```python
from build123d import *

# Parameters (mm, degrees)
SKETCH_W                        = 15
SKETCH_H                        = 25
PAD_DEPTH                       = 6
POCKET_DEPTH                    = 3
SKETCH002_R                     = 2.5
POCKET001_DEPTH                 = 3
SKETCH003_R                     = 1.5
POCKET002_DEPTH                 = 6.001
SKETCH004_R                     = 2
POCKET003_DEPTH                 = 1.5
SKETCH005_R                     = 1.5
POCKET004_DEPTH                 = 65.532504
SKETCH005_LINEARPATTERN_2_R     = 1.5
POCKET004_LINEARPATTERN_2_DEPTH = 65.532504
LINEARPATTERN001_COUNT          = 2
LINEARPATTERN001_PITCH          = 19
HOLE_D                          = 3
HOLE_DEPTH                      = 25
HOLE_CBORE_D                    = 5
HOLE_CBORE_DEPTH                = 1.5
FILLET_R                        = 1


with BuildPart() as part:
    # Sketch → Pad (new body)
    with BuildSketch(Plane.XY):
        Rectangle(SKETCH_W, SKETCH_H)
    extrude(amount=PAD_DEPTH)

    # Sketch001 (on Face6 of Pad) → Pocket (cut)
    with BuildSketch(Plane.XY.offset(6)):
        with BuildLine():
            Line((4, 4), (4, -4))
            ThreePointArc((-4, -4), (0, -8), (4, -4))
            Line((-4, -4), (-4, 4))
            ThreePointArc((4, 4), (0, 8), (-4, 4))
        make_face()
    extrude(amount=-POCKET_DEPTH, mode=Mode.SUBTRACT)

    # Sketch002 (on Face4 of Pocket) → Pocket001 (cut)
    with BuildSketch(Plane(origin=(0, 0, 0), x_dir=(1, 0, 0), z_dir=(0, 0, -1))):
        with Locations((4, 0)):
            Circle(SKETCH002_R)
    extrude(amount=-POCKET001_DEPTH, mode=Mode.SUBTRACT)

    # Sketch003 (on Face5 of Pocket001) → Pocket002 (cut, through all)
    with BuildSketch(Plane.XY.offset(6)):
        with Locations((4, 0)):
            Circle(SKETCH003_R)
    extrude(amount=-POCKET002_DEPTH, mode=Mode.SUBTRACT)

    # Sketch004 (on Face14 of Pocket002) → Pocket003 (cut)
    with BuildSketch(Plane.XY.offset(3)):
        with Locations((0, -4)):
            Circle(SKETCH004_R)
    extrude(amount=-POCKET003_DEPTH, mode=Mode.SUBTRACT)

    # Sketch005 (on Face5 of Pocket003) → Pocket004 (cut, through all)
    with BuildSketch(Plane.XY.offset(6)):
        with Locations((-4.5, 9.5)):
            Circle(SKETCH005_R)
    pocket004 = extrude(amount=-POCKET004_DEPTH, mode=Mode.SUBTRACT)

    # Sketch005 LinearPattern 2 → Pocket004 LinearPattern 2 (cut, through all)
    with BuildSketch(Plane(origin=(9, 0, 6), x_dir=(1, 0, 0), z_dir=(0, 0, 1))):
        with Locations((-4.5, 9.5)):
            Circle(SKETCH005_LINEARPATTERN_2_R)
    pocket004_linearpattern_2 = extrude(amount=-POCKET004_LINEARPATTERN_2_DEPTH, mode=Mode.SUBTRACT)

    # LinearPattern001: Pocket004, Pocket004 LinearPattern 2 ×2
    with Locations(*[(0, -i * LINEARPATTERN001_PITCH, 0) for i in range(1, LINEARPATTERN001_COUNT)]):
        add(pocket004, mode=Mode.SUBTRACT)
        add(pocket004_linearpattern_2, mode=Mode.SUBTRACT)

    # Hole
    with Locations(Plane(origin=(-7.5, 0, 0), x_dir=(0, -1, 0), z_dir=(-1, 0, 0))):
        with Locations((0, 3)):
            CounterBoreHole(HOLE_D / 2, HOLE_CBORE_D / 2, HOLE_CBORE_DEPTH, depth=HOLE_DEPTH)

    # Fillet
    fillet_edges = [part.edges().sort_by_distance(p)[0] for p in [
        (-7.5, -12.5, 3),
        (7.5, -12.5, 3),
        (-7.5, 12.5, 3),
        (7.5, 12.5, 3),
    ]]
    fillet(fillet_edges, radius=FILLET_R)


solid = part.part
```
Can you work these out from the model? Positions are in its coordinate system, mm. A direction names the side the tool comes from. Coordinates: 2 decimals unless noted, no trailing zeros. Loops run counter-clockwise (first coordinate to the right, second up) from the corner with the lowest first, then second, coordinate; pieces in that order, holes last.
Item 1: Suppose I cut it at B-B (x = -4.5). Please give me the cut outline in (y, z).
Answers below:
outline: (-12.5, 0) - (-11, 0) - (-11, 6) - (-12.5, 6) - close; (-8, 0) - (8, 0) - (8, 6) - (-8, 6) - close; (11, 0) - (12.5, 0) - (12.5, 6) - (11, 6) - close; hole circle Ø3 at (0, 3)
Item 2: Suppose I cut it at C-C (z = 3.5). State how many separate pieces and enclosed holes the cut face has, then the cut area to 3 significant figures.
Answers below:
separate pieces: 2
enclosed holes: 4
area: 209 mm2
Item 3: Suppose I cut it at A-A (y = -9.5). Please give me the cut outline in (x, z), then the cut area to 3 significant figures.
Answers below:
outline: (-7.5, 0) - (-6, 0) - (-6, 6) - (-7.5, 6) - close; (-3, 0) - (3, 0) - (3, 6) - (-3, 6) - close; (6, 0) - (7.5, 0) - (7.5, 6) - (6, 6) - close
area: 54.0 mm2
Item 4: Which directions (+Z, -Z, +X, -X, +Y, -Y) give clear straight access to the entire face, cutting with the end or side of a thin tool? Please do faces 5 (the face through (-2.833, -0.325, 1.536)), 6 (the face through (5, -2, 3)), 7 (the face through (5.5, 0, 4.9)), 8 (the face through (-7.215, -12.199, 3.042)), 9 (the face through (0, 5, 3)).
Answers below:
face 5: +X, -X
face 6: -Z
face 7: +Z, -Z
face 8: +Z, -Z, -X, -Y
face 9: +Z
Item 5: Please list where these lines run through material, in increasing order: L1, parallel to Y at x = 4.5, z = 4.2; L2, parallel to Y at x = -3.25, z = 2; L3, parallel to X at y = 2, z = 2.75.
Answers below:
L1: y = -12.5 to -11, -8 to -1.41, 1.41 to 8, 11 to 12.5
L2: y = -12.5 to -10.33, -8.67 to -1.12, 1.12 to 8.67, 10.33 to 12.5
L3: x = -6 to 2.5, 5.5 to 7.5
Item 6: I'm going to push flat-ended pins straight in: pin 1 (2 mm diameter, centred on x = 0, y = -4.5, fed in from +Z); pin 2 (4.5 mm diameter, centred on x = 0, y = -4, fed in from +Z). Where does each tip first touch, or does it pass through?
Answers below:
pin 1: stops at z = 1.5
pin 2: stops at z = 3
Item 7: If we mould it in two halves opening along Y, with no side actions, what happens to faces 1 (the face through (0, 12.5, 3)), 2 (the face through (6.163, -0.195, 4.487)), 3 (the face through (-7.5, -3, 3)), 4 (the face through (4, 3, 5))? For each: released by +Y, released by -Y, zero draft, split by the parting line, or undercut.
Answers below:
face 1: released by +Y
face 2: undercut
face 3: zero draft
face 4: undercut
Item 8: Suppose I cut it at D-D (y = 0). Please give me the cut outline in (x, z), then the cut area to 4 significant figures.
Answers below:
outline: (-7.5, 0) - (1.5, 0) - (1.5, 1.5) - (-6, 1.5) - (-6, 0.5) - (-7.5, 0.5) - close; (-7.5, 5.5) - (-6, 5.5) - (-6, 4.5) - (-4, 4.5) - (-4, 6) - (-7.5, 6) - close; (5.5, 4.5) - (7.5, 4.5) - (7.5, 6) - (5.5, 6) - close; (6.5, 0) - (7.5, 0) - (7.5, 1.5) - (6.5, 1.5) - close
area: 20.25 mm2
